```python
from build123d import *

# Parameters (mm, degrees)
SKETCH1_R           = 17.5
BOSS_EXTRUDE1_DEPTH = 3
SKETCH2_R           = 17.5
BOSS_EXTRUDE2_DEPTH = 0.5
SKETCH3_W           = 13.5
SKETCH3_H           = 13.5
SKETCH3_W_2         = 11.63
SKETCH3_H_2         = 11.63
SKETCH3_W_3         = 9.4
SKETCH3_H_3         = 9.4
BOSS_EXTRUDE3_DEPTH = 1.5
FILLET1_R           = 1
SKETCH4_R           = 17.5
CUT_EXTRUDE1_DEPTH  = 32.5
BOSS_EXTRUDE4_START = 3
SKETCH5_R           = 1
BOSS_EXTRUDE4_DEPTH = 3
SKETCH6_W           = 13.5
SKETCH6_H           = 13.5
BOSS_EXTRUDE6_DEPTH = 3
CHAMFER1_SIZE       = 0.1


with BuildPart() as part:
    # Sketch1 → Boss-Extrude1 (new body)
    with BuildSketch(Plane.XY):
        Circle(SKETCH1_R)
        with BuildLine():
            Line((-9.921567416, -1.25), (-14.021567416, -1.25))
            Line((-14.021567416, -1.25), (-14.021567416, 1.25))
            Line((-14.021567416, 1.25), (-9.921567416, 1.25))
            ThreePointArc((-9.921567416, 1.25), (0, 10), (9.921567416, 1.25))
            Line((9.921567416, 1.25), (14.021567416, 1.25))
            Line((14.021567416, 1.25), (14.021567416, -1.25))
            Line((14.021567416, -1.25), (9.921567416, -1.25))
            ThreePointArc((9.921567416, -1.25), (0, -10), (-9.921567416, -1.25))
        make_face(mode=Mode.SUBTRACT)
    extrude(amount=BOSS_EXTRUDE1_DEPTH)

    # Sketch2 → Boss-Extrude2 (add)
    with BuildSketch(Plane.XY.offset(3)):
        Circle(SKETCH2_R)
    extrude(amount=BOSS_EXTRUDE2_DEPTH)

    # Sketch3 → Boss-Extrude3 (add)
    # profile 1 of 2: a face of its own
    with BuildSketch(Plane.XY.offset(3.5)):
        Rectangle(SKETCH3_W, SKETCH3_H)
        Rectangle(SKETCH3_W_2, SKETCH3_H_2, mode=Mode.SUBTRACT)
    # profile 2 of 2: a face of its own
    with BuildSketch(Plane.XY.offset(3.5)):
        Rectangle(SKETCH3_W_3, SKETCH3_H_3)
    extrude(amount=BOSS_EXTRUDE3_DEPTH)

    # Fillet1
    fillet1_edges = [part.edges().sort_by_distance(p)[0] for p in [
        (4.7, 4.7, 4.25),
        (-4.7, 4.7, 4.25),
        (-4.7, -4.7, 4.25),
        (4.7, -4.7, 4.25),
        (5.815, -5.815, 4.25),
        (-5.815, -5.815, 4.25),
        (-5.815, 5.815, 4.25),
        (5.815, 5.815, 4.25),
    ]]
    fillet(fillet1_edges, radius=FILLET1_R)

    # Sketch4 → Cut-Extrude1 (cut)
    with BuildSketch(Plane(origin=(0, 0, 0), x_dir=(-1, 0, 0), z_dir=(0, 0, -1))):
        Circle(SKETCH4_R)
        with BuildLine():
            Line((-16, 3.2), (-16, -3.2))
            Line((-16, -3.2), (-12.083459769, -3.2))
            ThreePointArc((-12.083459769, -3.2), (0, -12.5), (12.083459769, -3.2))
            Line((12.083459769, -3.2), (16, -3.2))
            Line((16, -3.2), (16, 3.2))
            Line((16, 3.2), (12.083459769, 3.2))
            ThreePointArc((12.083459769, 3.2), (0, 12.5), (-12.083459769, 3.2))
            Line((-12.083459769, 3.2), (-16, 3.2))
        make_face(mode=Mode.SUBTRACT)
    extrude(amount=-CUT_EXTRUDE1_DEPTH, mode=Mode.SUBTRACT)

    # Sketch5 → Boss-Extrude4 (add)
    with BuildSketch(Plane.XY.offset(5).offset(BOSS_EXTRUDE4_START)):
        with Locations(Location((-3.7, 3.7, 0), (0, 0, 180))):
            Circle(SKETCH5_R)
        with Locations((3.7, 3.7)):
            Circle(SKETCH5_R)
        with Locations((3.7, -3.7)):
            Circle(SKETCH5_R)
        with Locations((-3.7, -3.7)):
            Circle(SKETCH5_R)
    extrude(amount=-BOSS_EXTRUDE4_DEPTH)

    # Sketch6 → Boss-Extrude6 (add)
    with BuildSketch(Plane.XY.offset(8)):
        Rectangle(SKETCH6_W, SKETCH6_H)
        with BuildLine():
            Line((-6.065, 4.815), (-6.065, -4.815))
            ThreePointArc((-6.065, -4.815), (-5.698883476, -5.698883476), (-4.815, -6.065))
            Line((-4.815, -6.065), (4.815, -6.065))
            ThreePointArc((4.815, -6.065), (5.698883476, -5.698883476), (6.065, -4.815))
            Line((6.065, -4.815), (6.065, 4.815))
            ThreePointArc((6.065, 4.815), (5.698883476, 5.698883476), (4.815, 6.065))
            Line((4.815, 6.065), (-4.815, 6.065))
            ThreePointArc((-4.815, 6.065), (-5.698883476, 5.698883476), (-6.065, 4.815))
        make_face(mode=Mode.SUBTRACT)
    extrude(amount=-BOSS_EXTRUDE6_DEPTH)

    # Chamfer1
    chamfer1_edges = [part.edges().sort_by_distance(p)[0] for p in [
        (-5.522106781, -5.522106781, 5),
        (5.522106781, 5.522106781, 5),
        (-5.522106781, 5.522106781, 5),
        (5.522106781, -5.522106781, 5),
        (-6.065, 0, 5),
        (-5.698883476, -5.698883476, 5),
        (0, -6.065, 5),
        (5.698883476, -5.698883476, 5),
        (6.065, 0, 5),
        (5.698883476, 5.698883476, 5),
        (0, 6.065, 5),
        (-5.698883476, 5.698883476, 5),
        (-5.815, 0, 5),
        (0, -5.815, 5),
        (5.815, 0, 5),
        (0, 5.815, 5),
    ]]
    chamfer(chamfer1_edges, length=CHAMFER1_SIZE)


solid = part.part
```
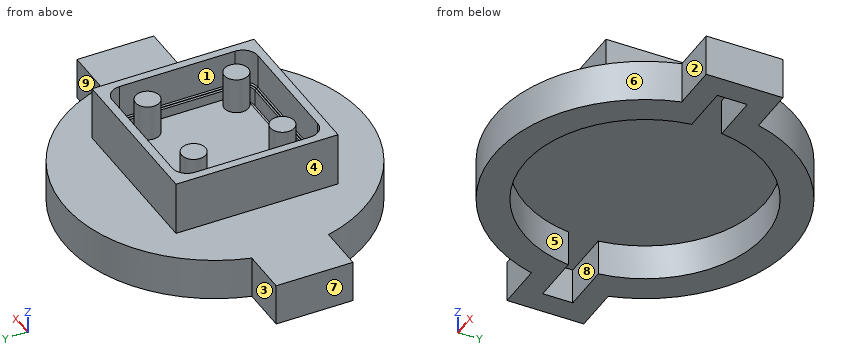
Work out the finished part from the listing and answer in its coordinate system (mm). Face numbers are marked on the shaded views. A direction names the side the tool comes from. Round coordinates to 2 decimals unless told otherwise and drop trailing zeros. Loops run counter-clockwise (first coordinate to the right, second up) from the corner with the lowest first, then second, coordinate; pieces in that order, holes last. Notation, with made-up numbers: (-15.75, 83) -> (2.25, 83) arc R31 cw to (2.25, 110) -> close; hole circle Ø9 at (-25.5, -20). An arc over 180 degrees is marked (long way). Write each question's results on one line, items separated by ' | '. Start each with the question number.
1. Find the intervals of material crossed by probe 1 along X at (y, z) = (2, 7.5) (3 decimals); probe 2 along Y at (x, z) = (-0.5, 3.75) (3 decimals), in increasing order. Write a range as from..to.
2. Section A-A (z = 6.75) is taken. Determine the outline of the cut face in (x, y) (3 decimals), plus the area to 3 significant figures.
3. Section D-D (y = -8.75) is taken. Determine the outline of the cut face in (x, z), plus the area to 3 significant figures.
4. A tool of negligible diameter and unlimited length cuts with its end or side. For the marked faces 1, 2, 3, 4 and 5, from which of +Z, -Z, +X, -X, +Y, -Y can it reach the whole face along a straight path? Write none if from no direction.
5. For a pull along Y with two mould halves and no side action, classify the marked faces 6, 7, 8 and 9 as +Y half, -Y half, draft (parallel to the pull), parting line (faces both ways), or undercut.
6. Given pin 1 Ø2 at (x, z) = (-6.5, 1) entering from -Y (3 decimals); pin 2 Ø1.3 at (x, z) = (1.5, 6) entering from +Y; pin 3 Ø1.5 at (x, z) = (-1.5, 7) entering from -Y, each flat-ended and moving along its own axis, determine where each tip first touches the part or whether it passes through.
7. Section C-C (x = -2) is taken. Determine the outline of the cut face in (y, z) (3 decimals).
Evaluation:
1) probe 1: x = -6.75..-6.065, 6.065..6.75 | probe 2: y = -6.75..-5.815, -4.7..4.7, 5.815..6.75
2) outline: (-6.75, -6.75) -> (6.75, -6.75) -> (6.75, 6.75) -> (-6.75, 6.75) -> close; circle Ø2 at (-3.7, -3.7); circle Ø2 at (-3.7, 3.7); circle Ø2 at (3.7, -3.7); circle Ø2 at (3.7, 3.7); hole (-6.065, -4.815) arc R1.25 ccw to (-4.815, -6.065) -> (4.815, -6.065) arc R1.25 ccw to (6.065, -4.815) -> (6.065, 4.815) arc R1.25 ccw to (4.815, 6.065) -> (-4.815, 6.065) arc R1.25 ccw to (-6.065, 4.815) -> close | area: 49.0 mm2
3) outline: (-8.93, 0) -> (-4.84, 0) -> (-4.84, 3) -> (4.84, 3) -> (4.84, 0) -> (8.93, 0) -> (8.93, 3.5) -> (-8.93, 3.5) -> close | area: 33.4 mm2
4) face 1: +Z | face 2: +Z, -Z, +X, -Y | face 3: +Z, -Z, -X, +Y | face 4: +Z, -X, +Y, -Y | face 5: -Z
5) face 6: -Y half | face 7: draft | face 8: undercut | face 9: +Y half
6) pin 1: stops at y = -11.225 | pin 2: stops at y = 6.75 | pin 3: stops at y = -6.75
7) outline: (-12.339, 0) -> (-9.798, 0) -> (-9.798, 3) -> (9.798, 3) -> (9.798, 0) -> (12.339, 0) -> (12.339, 3.5) -> (6.75, 3.5) -> (6.75, 8) -> (6.065, 8) -> (6.065, 5.1) -> (5.965, 5) -> (5.915, 5) -> (5.815, 4.9) -> (5.815, 3.5) -> (4.7, 3.5) -> (4.7, 5) -> (-4.7, 5) -> (-4.7, 3.5) -> (-5.815, 3.5) -> (-5.815, 4.9) -> (-5.915, 5) -> (-5.965, 5) -> (-6.065, 5.1) -> (-6.065, 8) -> (-6.75, 8) -> (-6.75, 3.5) -> (-12.339, 3.5) -> close
